Here's the drawing with two shaded views (mm, measured from the low corner). I have some questions. Coordinates: 2 decimals unless noted, no trailing zeros. Write each loop counter-clockwise with the first axis right and the second up, starting at its lowest first coordinate (ties: lowest second). Pieces come first, ordered by that corner, then holes. Notation, with made-up numbers: (53.25, 32.5) -> (89.25, 32.5) arc R19 ccw to (89.25, 39.5) -> close; hole circle Ø11 at (-12.75, 15.5). An arc over 180 degrees is marked (long way). Use a Markdown table: item, result. Add a question column.
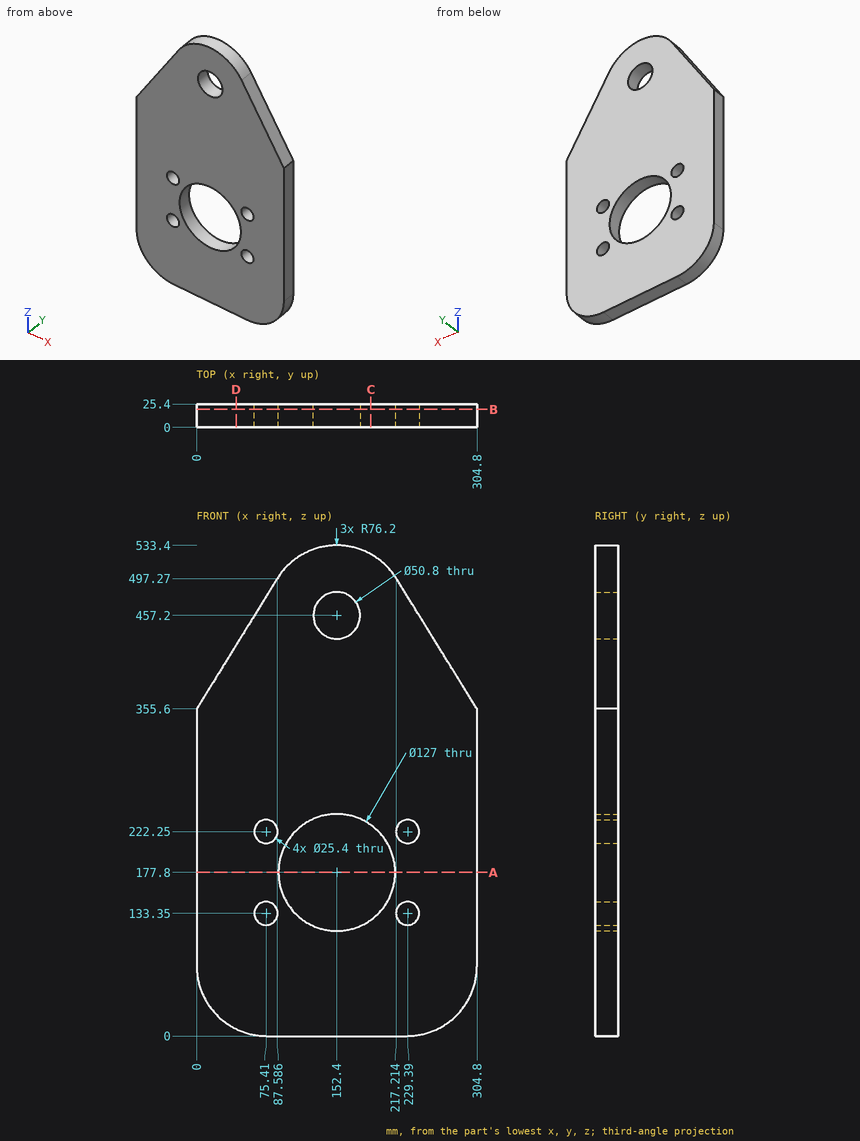
Q1. Suppose I cut it at A-A, the plane z = 177.8. Write out the boundary of the cut face in (x, y), and give its area (3 significant figures).
Q2. Suppose I cut it at C-C, the plane x = 189.5. Write out the boundary of the cut face in (y, z) (1 decimal), and give its area (3 significant figures).
Q3. Suppose I cut it at B-B, the plane y = 19.5. Write out the boundary of the cut face in (x, z), and give its area (3 significant figures).
Q4. Will these pins go through, and if not, where does the flat tip stop? pin 1 (15 mm diameter, centred on x = 75.41, z = 133.35, fed in from -Y); pin 2 (8 mm diameter, centred on x = 42, y = 5.5, fed in from -Z); pin 3 (1.5 mm diameter, centred on x = 125.5, y = 14.5, fed in from +Z); pin 4 (6 mm diameter, centred on y = 20.5, z = 362, fed in from -X).
Q5. Please list where these lines run through material, in increasing order: line 1 (Z direction, x = 152.4, y = 6.5); line 2 (Z direction, x = 76, y = 15) (1 decimal); line 3 (Z direction, x = 125, y = 21.5) (1 decimal).
Q6. Suppose I cut it at D-D, the plane x = 43. Write out the boundary of the cut face in (y, z), and give its area (3 significant figures).
Answer key:
| question | item | result |
|---|---|---|
| 1 | outline | (0, 0) -> (88.9, 0) -> (88.9, 25.4) -> (0, 25.4) -> close; (215.9, 0) -> (304.8, 0) -> (304.8, 25.4) -> (215.9, 25.4) -> close |
| 1 | area | 4,520 mm^2 |
| 2 | outline | (0, 0) -> (25.4, 0) -> (25.4, 126.3) -> (0, 126.3) -> close; (0, 229.3) -> (25.4, 229.3) -> (25.4, 523.8) -> (0, 523.8) -> close |
| 2 | area | 10,700 mm^2 |
| 3 | outline | (0, 76.2) arc R76.2 ccw to (76.2, 0) -> (228.6, 0) arc R76.2 ccw to (304.8, 76.2) -> (304.8, 355.6) -> (217.21, 497.27) arc R76.2 ccw to (87.59, 497.27) -> (0, 355.6) -> close; hole circle Ø25.4 at (75.41, 133.35); hole circle Ø25.4 at (75.41, 222.25); hole circle Ø127 at (152.4, 177.8); hole circle Ø50.8 at (152.4, 457.2); hole circle Ø25.4 at (229.39, 133.35); hole circle Ø25.4 at (229.39, 222.25) |
| 3 | area | 123,000 mm^2 |
| 4 | pin 1 | passes through |
| 4 | pin 2 | stops at z = 6.24 |
| 4 | pin 3 | stops at z = 528.77 |
| 4 | pin 4 | stops at x = 2.1 |
| 5 | line 1 | z = 0 to 114.3, 241.3 to 431.8, 482.6 to 533.4 |
| 5 | line 2 | z = 0 to 120.7, 146 to 209.6, 234.9 to 478.5 |
| 5 | line 3 | z = 0 to 120.5, 235.1 to 528.3 |
| 6 | outline | (0, 7.61) -> (25.4, 7.61) -> (25.4, 425.15) -> (0, 425.15) -> close |
| 6 | area | 10,600 mm^2 |
